For this review, use the dimensioned drawing (mm, ordinates from the lowest corner) and the shaded views. A direction names the side the tool comes from. Round coordinates to 2 decimals unless told otherwise and drop trailing zeros. Loops run counter-clockwise (first coordinate to the right, second up) from the corner with the lowest first, then second, coordinate; pieces in that order, holes last. Notation, with made-up numbers: (54.5, 79.25) -> (70.5, 79.25) arc R19 cw to (70.5, 96.25) -> close; hole circle Ø6 at (38, -21). An arc over 180 degrees is marked (long way). Use one line per item in the form item = value. Start each with the question number.
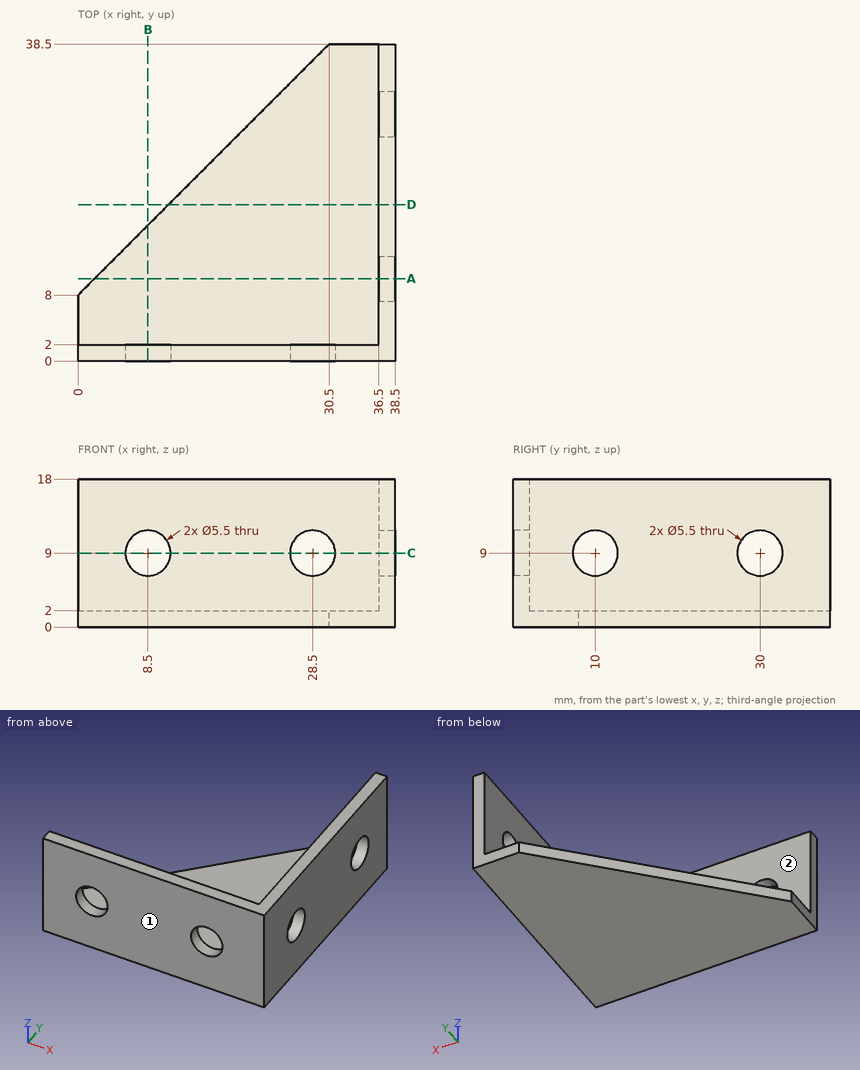
Item 1: Take a section at A-A on y = 10. Give the boundary of the cut face in (x, z), plus the area to 3 significant figures.
Item 2: For P1, Ø1.5, axis at y = 19, z = 8, coming from the -X side; P2, Ø9, axis at x = 8.5, z = 9, coming from the +Y side; P3, Ø11, axis at x = 18, y = 18, coming from the +Z side, all flat-tipped, find the tip position at first contact; note any pin that passes through.
Item 3: Machinability: for the marked faces 1 and 2, which of the approach directions +Z, -Z, +X, -X, +Y, -Y give a long, thin tool a straight path to every point of the face, cutting with its end or side? Answer none if there is none.
Item 4: Take a section at D-D on y = 19. Give the boundary of the cut face in (x, z), plus the area to 3 significant figures.
Item 5: Take a section at C-C on z = 9. Give the boundary of the cut face in (x, y).
Item 6: Wall thickness on line 1 (Y direction, x = 37.75, z = 9); line 2 (X direction, y = 1.2, z = 9); line 3 (Z direction, x = 34, y = 22.5): over which ranges is each line inside the solid? List them lowest first.
Item 7: Take a section at B-B on x = 8.5. Give the boundary of the cut face in (y, z), plus the area to 3 significant figures.
Results:
q1.outline = (2, 0) -> (38.5, 0) -> (38.5, 6.25) -> (36.5, 6.25) -> (36.5, 2) -> (2, 2) -> close; (36.5, 11.75) -> (38.5, 11.75) -> (38.5, 18) -> (36.5, 18) -> close
q1.area = 94.0 mm2
q2.P1 = 36.5
q2.P2 = 2
q2.P3 = 2
q3.face_1 = +Z, -Z, +X, -X, -Y
q3.face_2 = +Z, -X, +Y
q4.outline = (11, 0) -> (38.5, 0) -> (38.5, 18) -> (36.5, 18) -> (36.5, 2) -> (11, 2) -> close
q4.area = 87.0 mm2
q5.outline = (0, 0) -> (5.75, 0) -> (5.75, 2) -> (0, 2) -> close; (11.25, 0) -> (25.75, 0) -> (25.75, 2) -> (11.25, 2) -> close; (31.25, 0) -> (38.5, 0) -> (38.5, 7.25) -> (36.5, 7.25) -> (36.5, 2) -> (31.25, 2) -> close; (36.5, 12.75) -> (38.5, 12.75) -> (38.5, 27.25) -> (36.5, 27.25) -> close; (36.5, 32.75) -> (38.5, 32.75) -> (38.5, 38.5) -> (36.5, 38.5) -> close
q6.line_1 = 0 to 7.25, 12.75 to 27.25, 32.75 to 38.5
q6.line_2 = 0 to 5.75, 11.25 to 25.75, 31.25 to 38.5
q6.line_3 = 0 to 2
q7.outline = (0, 0) -> (16.5, 0) -> (16.5, 2) -> (2, 2) -> (2, 6.25) -> (0, 6.25) -> close; (0, 11.75) -> (2, 11.75) -> (2, 18) -> (0, 18) -> close
q7.area = 54.0 mm2
